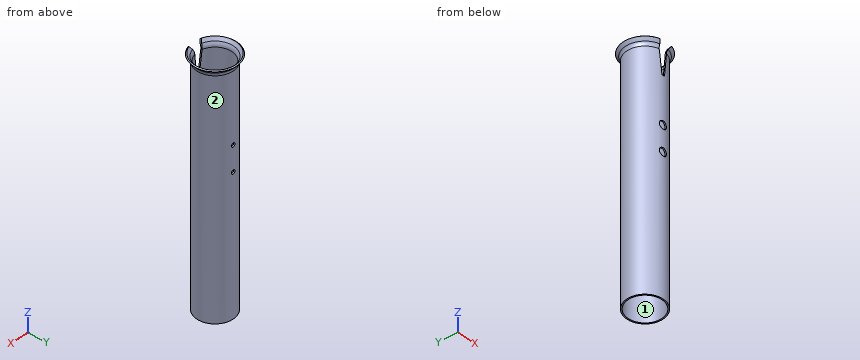
from build123d import *

# Parameters (mm, degrees)
F1_DEPTH      = 45
F3_DEPTH      = 47.5
F0_R          = 5
F0_R_2        = 2.5
F4_DEPTH      = 26.8448911594
F4_DEPTH_BACK = 10.2
F5_DEPTH      = 26.8448911594
F5_DEPTH_BACK = 17.3
F6_DEPTH      = 28.0842064241
F6_DEPTH_BACK = 25
F7_DEPTH      = 40.6
F7_DEPTH_BACK = 127.9
F8_DEPTH      = 26.8448911594
F8_DEPTH_BACK = 25


with BuildPart() as f1:
    # F0 (on Front) → F1 (new body)
    with BuildSketch(Plane.XZ):
        with BuildLine():
            ThreePointArc((-56.1564664539, 94.2714790144), (-55.7103223471, 94.4415023302), (-55.4904903386, 94.8653258548))
            Line((-55.4904903386, 94.8653258548), (-51.9799463815, 125.4227281117))
            ThreePointArc((-51.9799463815, 125.4227281117), (-50.9232927128, 129.1475665325), (-48.7355589867, 132.3420554399))
            Line((-48.7355589867, 132.3420554399), (-47.0069608027, 134.1516260741))
            Line((-47.0069608027, 134.1516260741), (-67.7195905025, 134.1516260741))
            Line((-67.7195905025, 134.1516260741), (-65.9909923185, 132.3420554399))
            ThreePointArc((-65.9909923185, 132.3420554399), (-63.8032585923, 129.1475665325), (-62.7466049237, 125.4227281117))
            Line((-62.7466049237, 125.4227281117), (-59.2360609666, 94.8653258548))
            ThreePointArc((-59.2360609666, 94.8653258548), (-59.0162289581, 94.4415023302), (-58.5700848513, 94.2714790144))
            Line((-58.5700848513, 94.2714790144), (-56.1564664539, 94.2714790144))
        make_face()
    extrude(amount=F1_DEPTH)

    # F0 (on Front) → F2 (revolve)
    with BuildSketch(Plane.XZ):
        with BuildLine():
            ThreePointArc((-33.5507006262, 129.2238042997), (-35.0548504452, 126.5545175576), (-35.5763814669, 123.535318362))
            Line((-35.5763814669, 123.535318362), (-35.5763814669, -173.2597642372))
            Line((-35.5763814669, -173.2597642372), (-33.9763798769, -173.2597642372))
            Line((-33.9763798769, -173.2597642372), (-33.9763798769, 123.535318362))
            ThreePointArc((-33.9763798769, 123.535318362), (-33.5475655735, 126.0177705006), (-32.3108204324, 128.2125169058))
            Line((-32.3108204324, 128.2125169058), (-29.2800693285, 131.9283431772))
            Line((-29.2800693285, 131.9283431772), (-30.5199495223, 132.9396305711))
            Line((-30.5199495223, 132.9396305711), (-33.5507006262, 129.2238042997))
        make_face()
    revolve(axis=Axis((-57.3632756526, 0, 129.4338501955), (0, 0, -1)))

    # F3 (cut): a face of the model
    f3_faces = [f1.faces().sort_by_distance(p)[0] for p in [
        (-57.3632756526, -45, 118.8376306589),
    ]]
    extrude(f3_faces, amount=-F3_DEPTH, mode=Mode.SUBTRACT)

    # F0 (on Front) → F4 (cut, two sides)
    with BuildSketch(Plane.XZ) as f4_sk:
        with Locations((-57.3632756526, 34.9645242095)):
            Circle(F0_R)
        with Locations((-57.3632756526, 34.9645242095)):
            Circle(F0_R_2, mode=Mode.SUBTRACT)
    extrude(amount=F4_DEPTH, mode=Mode.SUBTRACT)
    extrude(f4_sk.sketch, amount=-F4_DEPTH_BACK, mode=Mode.SUBTRACT)

    # F0 (on Front) → F5 (cut, two sides)
    with BuildSketch(Plane.XZ) as f5_sk:
        with Locations((-57.3632756526, 2.7531287633)):
            Circle(F0_R)
        with Locations((-57.3632756526, 2.7531287633)):
            Circle(F0_R_2, mode=Mode.SUBTRACT)
    extrude(amount=F5_DEPTH, mode=Mode.SUBTRACT)
    extrude(f5_sk.sketch, amount=-F5_DEPTH_BACK, mode=Mode.SUBTRACT)

    # F0 (on Front) → F6 (cut, two sides)
    with BuildSketch(Plane.XZ) as f6_sk:
        with Locations((-57.3632756526, 34.9645242095)):
            Circle(F0_R_2)
    extrude(amount=-F6_DEPTH, mode=Mode.SUBTRACT)
    extrude(f6_sk.sketch, amount=F6_DEPTH_BACK, mode=Mode.SUBTRACT)

    # F0 (on Front) → F7 (cut, two sides)
    with BuildSketch(Plane.XZ) as f7_sk:
        with Locations((-57.3632756526, 2.7531287633)):
            Circle(F0_R_2)
    extrude(amount=F7_DEPTH, mode=Mode.SUBTRACT)
    extrude(f7_sk.sketch, amount=-F7_DEPTH_BACK, mode=Mode.SUBTRACT)

    # F0 (on Front) → F8 (cut, two sides)
    with BuildSketch(Plane.XZ) as f8_sk:
        with Locations((-57.3632756526, 34.9645242095)):
            Circle(F0_R_2)
    extrude(amount=F8_DEPTH, mode=Mode.SUBTRACT)
    extrude(f8_sk.sketch, amount=-F8_DEPTH_BACK, mode=Mode.SUBTRACT)


solid = f1.part
Read the model definition and answer for the solid it produces. Units are mm, in the model's axes. Face numbers are marked on the shaded views. Round coordinates to 2 decimals unless told otherwise and drop trailing zeros. Order: outer loops, then holes, each group sorted by start corner. A loop starts at its lowest first (then second) coordinate and runs counter-clockwise, first axis right, second up.
1) Flat-ended cylindrical pins translate along their axes: pin 1 (2 mm diameter, centred on y = -19.5, z = 29.5, fed in from +X); pin 2 (9 mm diameter, centred on x = -57.36, z = 34.96, fed in from +Y); pin 3 (6 mm diameter, centred on x = -50, z = -25, fed in from -Y); pin 4 (4.5 mm diameter, centred on x = -57.36, z = 34.96, fed in from -Y). Find the tip coordinate at first contact, or state that the pin passes through.
2) The part is cut by section C-C on z = 103. Write down the section's boundary in (x, y).
3) The part is cut by section A-A on y = 0. Write down the section's boundary in (x, z), plus the area to 3 significant figures.
4) Straight lines are drawn through the part: L1, parallel to X at y = 0, z = 48; L2, parallel to Y at x = -42, z = 95.5. For each, find the intervals that lie inside material, in ascending order.
5) The mould has two halves that part along Y. Classify the marked faces 1 and 2: released by +Y, released by -Y, zero draft, split by the parting line, or undercut.
6) The part is cut by section B-B on z = -119.5. Write down the section's boundary in (x, y).
Resolved:
1. pin 1: stops at x = -43.06
1. pin 2: stops at y = 23.39
1. pin 3: stops at y = -22.98
1. pin 4: passes through
2. outline: (-60.17, -23.22) - (-60.17, -21.61) arc R21.79 cw (long way) to (-54.56, -21.61) - (-54.56, -23.22) arc R23.39 ccw (long way) to start
3. outline: (-85.45, 131.93) - (-82.42, 128.21) arc R7.4 cw to (-80.75, 123.54) - (-80.75, -173.26) - (-79.15, -173.26) - (-79.15, 123.54) arc R9 ccw to (-81.18, 129.22) - (-84.21, 132.94) - close; (-35.58, -173.26) - (-33.98, -173.26) - (-33.98, 123.54) arc R7.4 cw to (-32.31, 128.21) - (-29.28, 131.93) - (-30.52, 132.94) - (-33.55, 129.22) arc R9 ccw to (-35.58, 123.54) - close
3. area: 983 mm2
4. L1: x = -80.75 to -79.15, -35.58 to -33.98
4. L2: y = -17.63 to -15.45, 15.45 to 17.63
5. face 1: undercut
5. face 2: split by the parting line
6. outline: circle Ø46.77 at (-57.36, 0); hole circle Ø43.57 at (-57.36, 0)
